The listing builds one solid part. Answer for the finished solid, in the listing's coordinates (mm). A direction names the side the tool comes from. Give positions to 0.01 mm unless a question says otherwise; leave off trailing zeros. Order: outer loops, then holes, each group sorted by start corner. A loop starts at its lowest first (then second) coordinate and runs counter-clockwise, first axis right, second up. Notation, with made-up numbers: (27.5, 68.5) - (50.5, 68.5) arc R35 cw to (50.5, 107.5) - close; hole circle Ø8 at (86.5, -5). An arc over 180 degrees is marked (long way). Answer in a Markdown table with one row per item.
from build123d import *

# Parameters (mm, degrees)
BOSS_EXTRUDE1_DEPTH = 12.7
BOSS_EXTRUDE2_START = -3.583139
SKETCH3_W           = 9.863535196
SKETCH3_H           = 3.96875
BOSS_EXTRUDE2_DEPTH = 13.108139
FILLET1_R           = 1.905
CHAMFER1_SIZE       = 4.92
CHAMFER1_SIZE2      = 2.190525132
SKETCH5_W           = 4.064
SKETCH5_H           = 1.1176
CUT_EXTRUDE2_DEPTH  = 8.255


with BuildPart() as part:
    # Sketch1 → Boss-Extrude1 (new body)
    with BuildSketch(Plane.XY):
        Polygon((0, 0), (-4.931767598, 3.583138898), (-2.38125, 11.30060247), (2.38125, 11.30060247), (4.931767598, 3.583138898), align=None)
    extrude(amount=BOSS_EXTRUDE1_DEPTH)

    # Sketch3 → Boss-Extrude2 (add)
    with BuildSketch(Plane(origin=(0, 0, 0), x_dir=(-1, 0, 0), z_dir=(0, -1, 0)).offset(BOSS_EXTRUDE2_START)):
        with Locations((0, -6.35)):
            Rectangle(SKETCH3_W, SKETCH3_H)
    extrude(amount=BOSS_EXTRUDE2_DEPTH)

    # Fillet1
    fillet1_edges = [part.edges().sort_by_distance(p)[0] for p in [
        (-2.38125, 11.30060247, 6.35),
        (2.38125, 11.30060247, 6.35),
    ]]
    fillet(fillet1_edges, radius=FILLET1_R)

    # Chamfer1
    chamfer1_edges = [part.edges().sort_by_distance(p)[0] for p in [
        (4.931767598, -9.525, 6.35),
        (-4.931767598, -9.525, 6.35),
    ]]
    chamfer1_side = [part.faces().sort_by_distance(p)[0] for p in [
        (0, -9.525, 6.35),
    ]]
    chamfer(chamfer1_edges, length=CHAMFER1_SIZE, length2=CHAMFER1_SIZE2, reference=chamfer1_side[0])

    # Sketch5 → Cut-Extrude2 (cut)
    with BuildSketch(Plane(origin=(0, -9.525, 0), x_dir=(-1, 0, 0), z_dir=(0, -1, 0))):
        with Locations((0, -6.35)):
            Rectangle(SKETCH5_W, SKETCH5_H)
    extrude(amount=-CUT_EXTRUDE2_DEPTH, mode=Mode.SUBTRACT)


solid = part.part
Item 1: Find section C-C on x = 0.25. Write down the section's boundary in (y, z), then the cut area to 3 significant figures.
Answer block:
| item | result |
|---|---|
| outline | (-9.42, 4.37) - (0.18, 4.37) - (0.18, 0) - (11.3, 0) - (11.3, 12.7) - (0.18, 12.7) - (0.18, 8.33) - (-9.42, 8.33) - (-9.42, 6.91) - (-1.27, 6.91) - (-1.27, 5.79) - (-9.42, 5.79) - close |
| area | 170 mm² |
Item 2: Find section D-D on y = 1.25. Write down the section's boundary in (x, z).
Answer block:
| item | result |
|---|---|
| outline | (-4.93, 4.37) - (-1.72, 4.37) - (-1.72, 0) - (1.72, 0) - (1.72, 4.37) - (4.93, 4.37) - (4.93, 8.33) - (1.72, 8.33) - (1.72, 12.7) - (-1.72, 12.7) - (-1.72, 8.33) - (-4.93, 8.33) - close |
Item 3: Which of the six approach directions +Z, -Z, +X, -X, +Y, -Y give full straight-line access (tool end or side, diameter ignored) to faces 1 (the face through (-2.431, 1.766, 2.152)), 2 (the face through (0, -3, 4.366)), 3 (the face through (0, -1.27, 6))?
Answer block:
| item | result |
|---|---|
| face 1 | -Z, -X, -Y |
| face 2 | -Z, -Y |
| face 3 | -Y |
Item 4: Find section A-A on y = -2. Write down the section's boundary in (x, z).
Answer block:
| item | result |
|---|---|
| outline | (-4.93, 4.37) - (4.93, 4.37) - (4.93, 8.33) - (-4.93, 8.33) - close; hole (-2.03, 5.79) - (2.03, 5.79) - (2.03, 6.91) - (-2.03, 6.91) - close |
Item 5: Determine the mould class of faces 4 (the face through (-2.032, -5, 6)), 5 (the face through (0, 6, 0)), 6 (the face through (0, -5, 5.791)), 7 (the face through (3.86, 6.83, 6.26)) for opening direction Z: pulls with the +Z half, pulls with the -Z half, needs draft (parallel to the pull), parting line crosses it, or undercut.
Answer block:
| item | result |
|---|---|
| face 4 | undercut |
| face 5 | pulls with the -Z half |
| face 6 | undercut |
| face 7 | needs draft |
Item 6: Each of these flat-tipped pins is pushed along its axis until it touches: P1, Ø4, axis at x = 2, y = -4, coming from the +Z side; P2, Ø1.5, axis at x = 3, z = 6, coming from the +Y side; P3, Ø2, axis at y = 1, z = 8.5, coming from the +X side; P4, Ø5, axis at x = 2.5, y = -7, coming from the -Z side. Where does it stop, or does it pass through?
Answer block:
| item | result |
|---|---|
| P1 | z = 8.33 |
| P2 | y = 10.84 |
| P3 | x = 4.93 |
| P4 | z = 4.37 |
Item 7: Consider line 1 (Z direction, x = 0.5, y = -7); line 2 (Z direction, x = 3.75, y = 1.25); line 3 (Y direction, x = -2, z = 11.5). Determine where each line is inside the solid, lowest interval first.
Answer block:
| item | result |
|---|---|
| line 1 | 4.37 to 5.79, 6.91 to 8.33 |
| line 2 | 4.37 to 8.33 |
| line 3 | 1.45 to 11.02 |
Item 8: Find section B-B on z = 11. Write down the section's boundary in (x, y) (3 decimals).
Answer block:
| item | result |
|---|---|
| outline | (-4.932, 3.583) - (0, 0) - (4.932, 3.583) - (2.813, 9.993) arc R1.905 ccw to (1.004, 11.301) - (-1.004, 11.301) arc R1.905 ccw to (-2.813, 9.993) - close |
